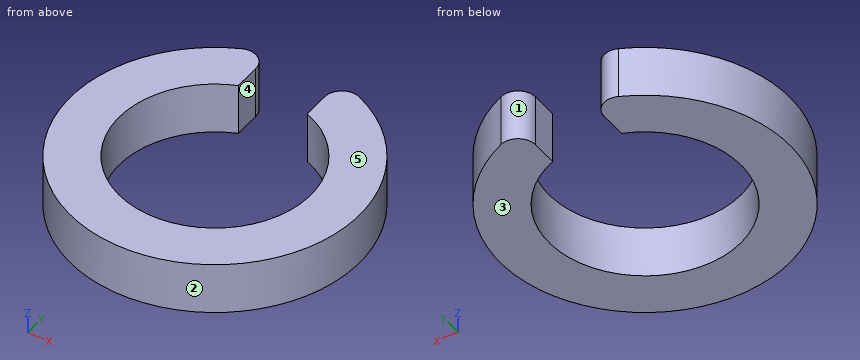
Autodesk Inventor part; units mm, degrees
ref_plane "YZ Plane" through (0, 0, 0) normal (1, 0, 0) x (0, 1, 0)
ref_plane "XZ Plane" through (0, 0, 0) normal (0, 1, 0) x (-1, 0, 0)
ref_plane "XY Plane" through (0, 0, 0) normal (0, 0, 1) x (1, 0, 0)
sketch "Sketch1" plane through (0, 0, 0) normal (0, 0, 1) x (1, 0, 0)
  circle A0 centre (0, 0) radius 5.55
  circle A1 centre (0, 0) radius 8.375
  line L0 (-2, 8.375) -> (2, 8.375)
  line L1 (2, 8.375) -> (2, 0)
  line L2 (2, 0) -> (-2, 0)
  line L3 (-2, 0) -> (-2, 8.375)
  point P0 (-2, 5.1771)
  point P1 (-2, 8.1327)
  point P2 (2, 8.1327)
  point P3 (2, 5.1771)
  dimension "d0" = 11.1
  dimension "d1" = 16.75
  dimension "d2" = 4
extrude "Extrusion1" add sketch "Sketch1" along normal blind 3 contours A0 L1 A1 L3 picked at (7.294, -1.1285)
fillet "Fillet1" radius 1 2 edges at (-2, 8.1327, 1.5) (2, 8.1327, 1.5)
properties part number "2002_Rx_Tx Coil Spacer_Glass_v3"
Work out the finished part from the listing and answer in its coordinate system (mm). Face numbers are marked on the shaded views. A direction names the side the tool comes from. Give positions to 0.01 mm unless a question says otherwise; leave off trailing zeros. Write each loop counter-clockwise with the first axis right and the second up, starting at its lowest first coordinate (ties: lowest second). Pieces come first, ordered by that corner, then holes. Notation, with made-up numbers: M 66.25,22.5 L 117.25,22.5 A31 cw 117.25,53.5 Z; hole C 61,18.5 d2. An arc over 180 degrees is marked long. Answer as CSV lines item,"result".
Q1. The mould has two halves that part along X. Classify the marked faces 1, 2 and 3: +X half, -X half, draft (parallel to the pull), parting line (faces both ways), or undercut.
A:
face 1,"undercut"
face 2,"parting line"
face 3,"draft"
Q2. A cutting plane is placed at C-C on x = 0. Write down the section's boundary in (y, z) (3 decimals), plus the area to 4 significant figures.
A:
outline,"M -8.375,0 L -5.55,0 L -5.55,3 L -8.375,3 Z"
area,"8.475 mm²"
Q3. A cutting plane is placed at D-D on y = 5.75. Write down the section's boundary in (x, z).
A:
outline,"M -6.09,0 L -2,0 L -2,3 L -6.09,3 Z; M 2,0 L 6.09,0 L 6.09,3 L 2,3 Z"
Q4. A cutting plane is placed at A-A on y = 0. Write down the section's boundary in (x, z) (3 decimals).
A:
outline,"M -8.375,0 L -5.55,0 L -5.55,3 L -8.375,3 Z; M 5.55,0 L 8.375,0 L 8.375,3 L 5.55,3 Z"
Q5. A cutting plane is placed at B-B on z = 2.8. Write down the section's boundary in (x, y) (3 decimals).
A:
outline,"M -3.407,7.651 A8.375 ccw long 3.407,7.651 A1 ccw 2,6.737 L 2,5.177 A5.55 cw long -2,5.177 L -2,6.737 A1 ccw Z"
Q6. A tool of negligible diameter and unlimited length cuts with its end or side. For the marked faces 4 and 5, from which of +Z, -Z, +X, -X, +Y, -Y can it reach the whole face along a straight path? Write none if from no direction.
A:
face 4,"+Z, -Z, +Y"
face 5,"+Z, +X, -X, +Y, -Y"
Q7. Given P1, Ø1.5, axis at x = 6, z = 0.5, coming from the -Y side; P2, Ø5, axis at x = 3, y = 2.5, coming from the +Z side; P3, Ø0.8, axis at y = 6, z = 1, coming from the +X side; P4, Ø0.8, axis at y = 6, z = 1, coming from the -X side, each flat-ended and moving along its own axis, determine where each tip first touches the part or whether it passes through.
A:
P1,"stops at y = -6.53"
P2,"stops at z = 3"
P3,"stops at x = 6.23"
P4,"stops at x = -6.23"
Q8. Find the intervals of material crossed by probe 1 along X at (y, z) = (0, 1.9) (3 decimals); probe 2 along Y at (x, z) = (0, 0.1) (3 decimals); probe 3 along Y at (x, z) = (2.5, 1.6), in increasing order. Write a range as [from, to].
A:
probe 1,"x = [-8.375, -5.55], [5.55, 8.375]"
probe 2,"y = [-8.375, -5.55]"
probe 3,"y = [-7.99, -4.96], [4.96, 7.6]"
